from build123d import *

# Parameters (mm, degrees)
IZIM1_R                     = 8
Y_KSEKLIK_EKSTR_ZYON1_DEPTH = 100
RADYUS1_R                   = 0.5
IZIM4_W                     = 7.745966692
IZIM4_H                     = 1
KES_EKSTR_ZYON2_DEPTH       = 8
CORTAR_EXTRUIR1_DEPTH       = 101.637965119
CORTAR_EXTRUIR1_DEPTH_BACK  = 101.637965119
CROQUIS1_R                  = 4.579234369


with BuildPart() as part:
    # Çizim1 → Yükseklik-Ekstrüzyon1 (new body)
    with BuildSketch(Plane.XY):
        Circle(IZIM1_R)
    extrude(amount=Y_KSEKLIK_EKSTR_ZYON1_DEPTH)

    # Radyus1
    radyus1_edges = [part.edges().sort_by_distance(p)[0] for p in [
        (-8, 0, 100),
    ]]
    fillet(radyus1_edges, radius=RADYUS1_R)

    # Çizim3 → M5x0.8 Tapped Hole1 (revolve, cut)
    with BuildSketch(Plane(origin=(0, 0, 100), x_dir=(0, -1, 0), z_dir=(1, 0, 0))):
        Polygon((0, 0), (0, 23.6618073), (2.1, 22.4), (2.1, 0), align=None)
    revolve(axis=Axis((0, 0, 106.35), (0, 0, -1)), mode=Mode.SUBTRACT)

    # Çizim4 → Kes-Ekstrüzyon2 (cut)
    with BuildSketch(Plane.XY.offset(100)):
        with Locations((0, 7.5)):
            Rectangle(IZIM4_W, IZIM4_H)
    extrude(amount=-KES_EKSTR_ZYON2_DEPTH, mode=Mode.SUBTRACT)

    # Croquis1 → Cortar-Extruir1 (cut, two sides: drawn at the far end of the back side and taken through both)
    with BuildSketch(Plane(origin=(0, 0, 0), x_dir=(1, 0, 0), z_dir=(0, 1, 0)).offset(-CORTAR_EXTRUIR1_DEPTH_BACK)):
        with Locations(Location((0, -92, 0), (0, 0, 270))):
            Circle(CROQUIS1_R)
    extrude(amount=CORTAR_EXTRUIR1_DEPTH + CORTAR_EXTRUIR1_DEPTH_BACK, mode=Mode.SUBTRACT)


solid = part.part
Source: CAD feature listing. Evaluate the final solid. Frame: model axes, mm. A direction names the side the tool comes from. Give positions to 0.01 mm unless a question says otherwise; leave off trailing zeros. Write each loop counter-clockwise with the first axis right and the second up, starting at its lowest first coordinate (ties: lowest second). Pieces come first, ordered by that corner, then holes. Notation, with made-up numbers: (11, -6) -> (63, -6) arc R21 cw to (63, 14) -> close; hole circle Ø8 at (-36, 30). An arc over 180 degrees is marked (long way). Write item = value, one per line.
Q1. First-contact query: pin 1 (4.5 mm diameter, centred on x = 0.5, z = 97, fed in from +Y); pin 2 (8 mm diameter, centred on y = -5.5, z = 37, fed in from -X); pin 3 (1 mm diameter, centred on x = 6, z = 37, fed in from -Y). Flat tips, straight axial feed; report the tip coordinate or a pass-through.
Here are the results:
pin_1 = 7
pin_2 = -7.86
pin_3 = -5.81
Q2. Line query: line 1 (X direction, y = 0, z = 98.85); line 2 (Z direction, x = 0, y = -4.5); line 3 (Y direction, x = 0, z = 97.55). Output: solid intervals per line, ascending. Write a range as from..to.
Here are the results:
line_1 = -8..-2.1, 2.1..8
line_2 = 0..87.42, 96.58..100
line_3 = -8..-2.1, 2.1..7
Q3. Cut plane A-A on z = 85. Return loops of the section in (x, y).
Here are the results:
outline = circle Ø16 at (0, 0); hole circle Ø4.2 at (0, 0)
Q4. Mould query, pull axis X, two halves, no side actions, for faces 4 (the face through (0, 0, 0)), 5 (the face through (-8, 0, 49)), 6 (the face through (-0.631, -2.003, 82.838)). Classes: +X half, -X half, draft (parallel to the pull), parting line (faces both ways), or undercut.
Here are the results:
face_4 = draft
face_5 = parting line
face_6 = undercut
Q5. Reachability of faces 1 (the face through (0, 7, 98)), 2 (the face through (2, -2, 100)), 3 (the face through (-0.631, -2.003, 98.062)) from +Z, -Z, +X, -X, +Y, -Y: full face, straight path, thin tool, end or side. Return the list, or none.
Here are the results:
face_1 = +Z, +X, -X, +Y
face_2 = +Z, +X, -X, +Y, -Y
face_3 = +Z
Q6. Cut plane B-B on z = 31.5. Return loops of the section in (x, y).
Here are the results:
outline = circle Ø16 at (0, 0)
